Work out the finished part from the listing and answer in its coordinate system (mm). Face numbers are marked on the shaded views. A direction names the side the tool comes from. Round coordinates to 2 decimals unless told otherwise and drop trailing zeros. Write each loop counter-clockwise with the first axis right and the second up, starting at its lowest first coordinate (ties: lowest second). Pieces come first, ordered by that corner, then holes.
1. Find section B-B (y = 39). Write down the section's boundary in (x, z).
2. Find section D-D (y = -27). Write down the section's boundary in (x, z).
3. Determine the mould class of the marked faces 4, 5 and 6 for opening direction Y: pulls with the +Y half, pulls with the -Y half, needs draft (parallel to the pull), parting line crosses it, or undercut.
4. Flat-ended cylindrical pins translate along their axes: pin 1 Ø9 at (y, z) = (22.5, -1) entering from +X; pin 2 Ø21.5 at (y, z) = (-31, -3) entering from -X; pin 3 Ø13 at (x, z) = (-0.5, -0.5) entering from -Y. Find the tip coordinate at first contact, or state that the pin passes through.
5. Straight lines are drawn through the part: probe 1 along X at (y, z) = (34.5, -1); probe 2 along Y at (x, z) = (-7.5, -12); probe 3 along X at (y, z) = (22.5, 4). For each, find the intervals that lie inside material, in ascending order.
6. A tool of negligible diameter and unlimited length cuts with its end or side. For the marked faces 1, 2 and 3, from which of +Z, -Z, +X, -X, +Y, -Y can it reach the whole face along a straight path? Write none if from no direction.
7. Find section C-C (x = 6). Write down the section's boundary in (y, z).
```python
from build123d import *

# Parameters (mm, degrees)
F1_DEPTH = 21
F2_W     = 10
F2_H     = 28
F3_DEPTH = 75.001
F4_W     = 16
F4_H     = 34
F5_DEPTH = 42.001
F6_W     = 7
F6_H     = 20
F7_DEPTH = 14


with BuildPart() as f1:
    # F0 (on Top) → F1 (new body, symmetric)
    with BuildSketch(Plane.XY):
        with BuildLine():
            Line((-8, -28), (0, -28))
            Line((0, -28), (8, -28))
            Line((8, -28), (8, -47))
            Line((8, -47), (18, -47))
            Line((18, -47), (18, -20.124612))
            ThreePointArc((18, -20.124612), (24.647515, -11.022704), (27, 0))
            ThreePointArc((27, 0), (24.647515, 11.022704), (18, 20.124612))
            Line((18, 20.124612), (18, 47))
            Line((18, 47), (8, 47))
            Line((8, 47), (8, 28))
            Line((8, 28), (0, 28))
            Line((0, 28), (-8, 28))
            Line((-8, 28), (-8, 47))
            Line((-8, 47), (-18, 47))
            Line((-18, 47), (-18, 20.124612))
            ThreePointArc((-18, 20.124612), (-24.647515, 11.022704), (-27, 0))
            ThreePointArc((-27, 0), (-24.647515, -11.022704), (-18, -20.124612))
            Line((-18, -20.124612), (-18, -47))
            Line((-18, -47), (-8, -47))
            Line((-8, -47), (-8, -28))
        make_face()
    extrude(amount=F1_DEPTH, both=True)

    # F2 (on face) → F3 (cut, through all)
    with BuildSketch(Plane.XZ.offset(28)):
        Rectangle(F2_W, F2_H)
    extrude(amount=-F3_DEPTH, mode=Mode.SUBTRACT)

    # F4 (on face) → F5 (cut, through all)
    with BuildSketch(Plane.XY.offset(21)):
        Rectangle(F4_W, F4_H)
    extrude(amount=-F5_DEPTH, mode=Mode.SUBTRACT)

    # F6 (on face) → F7 (cut)
    with BuildSketch(Plane.XY.offset(21)):
        with Locations((-11.5, 0)):
            Rectangle(F6_W, F6_H)
    extrude(amount=-F7_DEPTH, mode=Mode.SUBTRACT)


solid = f1.part
```
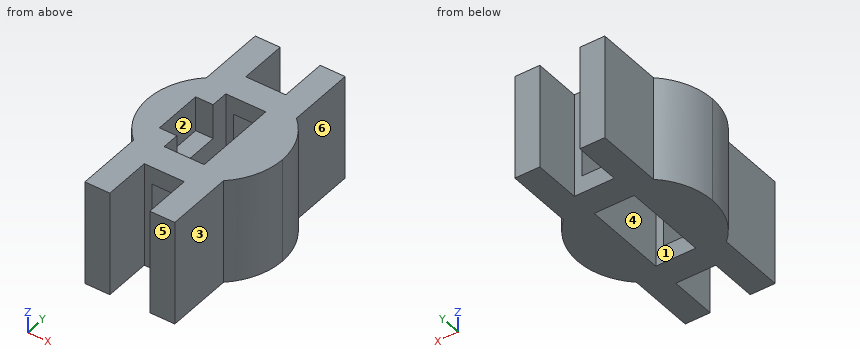
Worked answers:
1. outline: (-18, -21) - (-8, -21) - (-8, 21) - (-18, 21) - close; (8, -21) - (18, -21) - (18, 21) - (8, 21) - close
2. outline: (-18, -21) - (18, -21) - (18, 21) - (-18, 21) - close; hole (-5, -14) - (5, -14) - (5, 14) - (-5, 14) - close
3. face 4: undercut
3. face 5: pulls with the -Y half
3. face 6: needs draft
4. pin 1: stops at x = 20.12
4. pin 2: stops at x = -18
4. pin 3: stops at y = -28
5. probe 1: x = -18 to -8, 8 to 18
5. probe 2: y = -28 to -17, 17 to 28
5. probe 3: x = -18 to -5, 5 to 18
6. face 1: +Z, -Z
6. face 2: +Z
6. face 3: +Z, -Z, +X, -Y
7. outline: (-28, -21) - (-17, -21) - (-17, 21) - (-28, 21) - close; (17, -21) - (28, -21) - (28, 21) - (17, 21) - close
